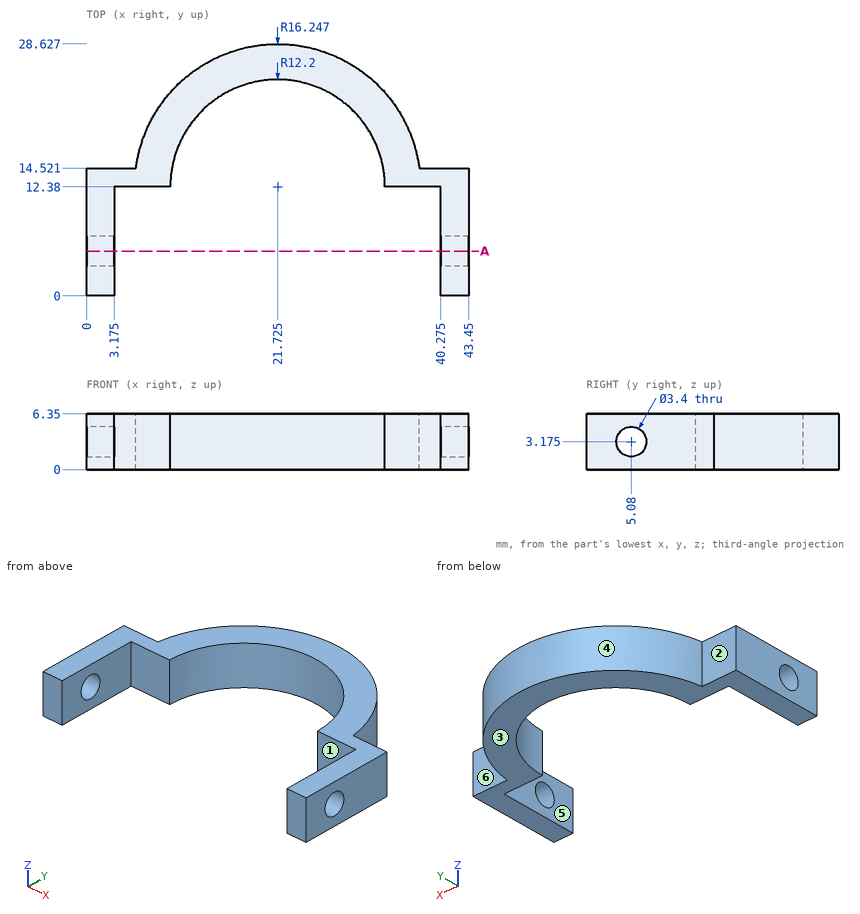
Could you check a few things on this drawing? It's one solid part, dimensions in mm from its lowest x, y, z. A direction names the side the tool comes from. Coordinates: 2 decimals unless noted, no trailing zeros. Answer as a JSON object with one key per item and string values. Group by question number.
Q1. I need wall thicknesses on line 1 (Y direction, x = 41.5, z = 3); line 2 (Y direction, x = 38, z = 0.75); line 3 (Y direction, x = 22, z = 1.75). Which ranges of each line are inside material? Lowest first, please. Write a range as from..to.
Q2. Will these pins go through, and if not, where does the flat tip stop? P1, Ø2, axis at x = 36, z = 2.5, coming from the -Y side; P2, Ø1, axis at x = 30, z = 2.5, coming from the +Y side (1 decimal); P3, Ø1, axis at x = 31.5, z = 2, coming from the +Y side; P4, Ø2, axis at y = 5.08, z = 3.175, coming from the -X side.
Q3. On a 3-axis mill with a long thin cutter (end or side, diameter ignored), from which of +Z, -Z, +X, -X, +Y, -Y can I reach the whole of each face in a straight line? I mean the marked faces 1, 2 and 3. Say none if no direction works.
Q4. Imagine slicing it at A-A (y = 5.08). Give the number of separate pieces and of enclosed holes in the cut face.
Q5. We'd pull the mould along X, two halves only. Please class the marked faces 4, 5 and 6: +X half, -X half, draft (parallel to the pull), parting line (faces both ways), or undercut.
Determined:
{
 "1": {"line 1": "y = 0..3.39, 6.77..14.52", "line 2": "y = 12.38..14.52", "line 3": "y = 24.58..28.62"},
 "2": {"P1": "stops at y = 12.38", "P2": "stops at y = 26.6", "P3": "stops at y = 25.72", "P4": "passes through"},
 "3": {"face 1": "+Z, -Z, -Y", "face 2": "+Z, -Z, -X, +Y", "face 3": "-Z, +X, -X, +Y, -Y"},
 "4": {"separate pieces": "4", "enclosed holes": "0"},
 "5": {"face 4": "parting line", "face 5": "undercut", "face 6": "draft"}
}
